Read the model definition and answer for the solid it produces. Units are mm, in the model's axes. A direction names the side the tool comes from. Coordinates: 2 decimals unless noted, no trailing zeros. Write each loop counter-clockwise with the first axis right and the second up, starting at its lowest first coordinate (ties: lowest second). Pieces come first, ordered by that corner, then holes. Notation, with made-up numbers: M 84.25,78 L 129.25,78 A19 cw 129.25,106 Z; hole C 27.25,86 d6. An arc over 180 degrees is marked long. Write item = value, one per line.
from build123d import *

# Parameters (mm, degrees)
ESQUISSE1_R             = 37.5
EXTRUSION1_DEPTH        = 5
ENL_V_MAT_EXTRU_2_DEPTH = 2.5
ESQUISSE7_R             = 7.5
ENL_V_MAT_EXTRU_3_DEPTH = 54.091901454
TROU_TARAUD_M4X0_71_D   = 3.3


with BuildPart() as part:
    # Esquisse1 → Extrusion1 (new body)
    with BuildSketch(Plane(origin=(0, 0, 0), x_dir=(1, 0, 0), z_dir=(0, 1, 0))):
        with Locations(Location((0, 0, 0), (0, 0, 270))):
            Circle(ESQUISSE1_R)
    extrude(amount=-EXTRUSION1_DEPTH)

    # Esquisse6 → Enlèv. mat.-Extru.2 (cut)
    with BuildSketch(Plane.XZ.offset(5)):
        with BuildLine():
            Line((-9.95, 1), (-9.95, -21.8))
            ThreePointArc((-9.95, -21.8), (-7.313961031, -28.163961031), (-0.95, -30.8))
            Line((-0.95, -30.8), (0.95, -30.8))
            ThreePointArc((0.95, -30.8), (7.313961031, -28.163961031), (9.95, -21.8))
            Line((9.95, -21.8), (9.95, 1))
            ThreePointArc((9.95, 1), (7.313961031, 7.363961031), (0.95, 10))
            Line((0.95, 10), (-0.95, 10))
            ThreePointArc((-0.95, 10), (-7.313961031, 7.363961031), (-9.95, 1))
        make_face()
    extrude(amount=-ENL_V_MAT_EXTRU_2_DEPTH, mode=Mode.SUBTRACT)

    # Esquisse7 → Enlèv. mat.-Extru.3 (cut, through all)
    with BuildSketch(Plane.XZ.offset(2.5)):
        Circle(ESQUISSE7_R)
    extrude(amount=-ENL_V_MAT_EXTRU_3_DEPTH, mode=Mode.SUBTRACT)

    # Trou taraudé M4x0.71 (through all)
    with Locations(Plane.XZ.offset(5)):
        with Locations((-5, -34.4), (5, -34.4), (-5, 13.6), (5, 13.6), (22.5, 0), (-22.5, 0)):
            Hole(TROU_TARAUD_M4X0_71_D / 2)


solid = part.part
Item 1: Find section C-C (x = 5). Determine the outline of the cut face in (y, z).
Worked answers:
outline = M -5,-37.17 L 0,-37.17 L 0,-36.05 L -5,-36.05 Z; M -5,-32.75 L 0,-32.75 L 0,-5.59 L -2.5,-5.59 L -2.5,-29.84 L -5,-29.84 Z; M -5,9.04 L -2.5,9.04 L -2.5,5.59 L 0,5.59 L 0,11.95 L -5,11.95 Z; M -5,15.25 L 0,15.25 L 0,37.17 L -5,37.17 Z
Item 2: Find section A-A (x = 22.5). Determine the outline of the cut face in (y, z).
Worked answers:
outline = M -5,-30 L 0,-30 L 0,-1.65 L -5,-1.65 Z; M -5,1.65 L 0,1.65 L 0,30 L -5,30 Z
Item 3: Find section B-B (z = 0). Determine the outline of the cut face in (x, y).
Worked answers:
outline = M -37.5,-5 L -24.15,-5 L -24.15,0 L -37.5,0 Z; M -20.85,-5 L -9.95,-5 L -9.95,-2.5 L -7.5,-2.5 L -7.5,0 L -20.85,0 Z; M 7.5,-2.5 L 9.95,-2.5 L 9.95,-5 L 20.85,-5 L 20.85,0 L 7.5,0 Z; M 24.15,-5 L 37.5,-5 L 37.5,0 L 24.15,0 Z
Item 4: For a pull along Z with two mould halves and no side action, classify faces 1 (the face through (-8, -5, 8)), 2 (the face through (7.384, -3.768, 7.294)) as released by +Z, released by -Z, zero draft, split by the parting line, or undercut.
Worked answers:
face_1 = zero draft
face_2 = undercut
Item 5: Which of the six approach directions +Z, -Z, +X, -X, +Y, -Y give full straight-line access (tool end or side, diameter ignored) to faces 3 (the face through (-7.384, -3.768, -28.094)), 4 (the face through (5.4, -2.5, 12))?
Worked answers:
face_3 = -Y
face_4 = +Y, -Y
Item 6: Flat-ended cylindrical pins translate along their axes: pin 1 (10 mm diameter, centred on x = -4, z = -3, fed in from -Y); pin 2 (8 mm diameter, centred on x = 16, z = 10.5, fed in from +Y); pin 3 (0.8 mm diameter, centred on y = -4, z = -14.5, fed in from +X); pin 4 (3 mm diameter, centred on y = -2, z = 7.5, fed in from +X). Find the tip coordinate at first contact, or state that the pin passes through.
Worked answers:
pin_1 = -2.5
pin_2 = 0
pin_3 = 34.75
pin_4 = 37.02
Item 7: Consider line 1 along Z through (x, y) = (-5, -3.6); line 2 along Z through (x, y) = (-5, -1.55); line 3 along Y through (x, z) = (-1.5, -8). Determine where each line is inside the solid, lowest interval first. Write a range as from..to.
Worked answers:
line_1 = -37.17..-36.05, -32.75..-29.84, 9.04..11.95, 15.25..37.17
line_2 = -37.17..-36.05, -32.75..-5.59, 5.59..11.95, 15.25..37.17
line_3 = -2.5..0
Item 8: Find section D-D (y = -0.9). Determine the outline of the cut face in (x, z), and give its area (3 significant figures).
Worked answers:
outline = C 0,0 d75; hole C -22.5,0 d3.3; hole C 0,0 d15; hole C -5,-34.4 d3.3; hole C -5,13.6 d3.3; hole C 5,-34.4 d3.3; hole C 5,13.6 d3.3; hole C 22.5,0 d3.3
area = 4,190 mm²
